Check sheet for the modelled part. Datum: model origin and axes. Units: mm. Face numbers are marked on the shaded views. A direction names the side the tool comes from. Round coordinates to 2 decimals unless told otherwise and drop trailing zeros. Write each loop counter-clockwise with the first axis right and the second up, starting at its lowest first coordinate (ties: lowest second). Pieces come first, ordered by that corner, then holes.
Item 1: Set-up check for the marked faces 1 and 2: record each of +Z, -Z, +X, -X, +Y, -Y from which the full face is reachable in a straight line by a thin tool's end or side.
Item 2: Release check for a two-part mould opening along Z. For the marked faces 3, 4 and 5 record: pulls with the +Z half, pulls with the -Z half, needs draft (parallel to the pull), parting line crosses it, or undercut.
Item 3: Section check B-B, the plane y = 182. Record the cut outline in (x, z), plus the area to 3 significant figures.
Item 4: Material ranges on line 1 along Y through (x, z) = (242.5, 232); line 2 along X through (y, z) = (-184, 194); line 3 along Z through (x, y) = (193.5, 17), recorded low to high.
Item 5: Section check A-A, the plane z = 388.5. State how many separate pieces and enclosed holes the cut face has, plus the area to 3 significant figures.
Item 6: Depth check by flat-ended pin: pin 1 (5 mm diameter, centred on x = 107, y = 40.5, fed in from -Z). Enter the tip coordinate at first touch or a pass-through.
Item 7: Section check C-C, the plane x = 253.5. Record the cut outline in (y, z).
from build123d import *

# Parameters (mm, degrees)
F0_W      = 600
F0_H      = 900
F1_DEPTH  = 500
F2_W      = 475
F2_H      = 150
F3_DEPTH  = 1705
F4_W      = 475
F4_H      = 280
F5_DEPTH  = 846
F6_W      = 100
F6_H      = 500
F7_DEPTH  = 63
F8_DEPTH  = 63
F9_DEPTH  = 63
F10_DEPTH = 63
F11_DEPTH = 63
F13_W     = 100
F13_H     = 500
F14_DEPTH = 63
F15_DEPTH = 63
F16_DEPTH = 63


with BuildPart() as f1:
    # F0 (on Top) → F1 (new body)
    with BuildSketch(Plane.XY):
        Rectangle(F0_W, F0_H)
    extrude(amount=F1_DEPTH)

    # F2 (on face) → F3 (cut)
    with BuildSketch(Plane.XZ.offset(450)):
        with Locations((0, 75)):
            Rectangle(F2_W, F2_H)
    extrude(amount=-F3_DEPTH, mode=Mode.SUBTRACT)

    # F4 (on face) → F5 (cut)
    with BuildSketch(Plane.XZ.offset(450)):
        with Locations((0, 330)):
            Rectangle(F4_W, F4_H)
    extrude(amount=-F5_DEPTH, mode=Mode.SUBTRACT)

    # F6 (on face) → F7 (cut)
    with BuildSketch(Plane.YZ.offset(300)):
        with Locations((-25, 250)):
            Rectangle(F6_W, F6_H)
    extrude(amount=-F7_DEPTH, mode=Mode.SUBTRACT)

    # F8 (add): a face of the model
    f8_faces = [f1.faces().sort_by_distance(p)[0] for p in [
        (237, -25, 485),
    ]]
    extrude(f8_faces, amount=F8_DEPTH)

    # F9 (add): a face of the model
    f9_faces = [f1.faces().sort_by_distance(p)[0] for p in [
        (237, -25, 170),
    ]]
    extrude(f9_faces, amount=F9_DEPTH)

    # F6 (on face) → F10 (cut)
    with BuildSketch(Plane.YZ.offset(300)):
        with Locations((325, 250)):
            Rectangle(F6_W, F6_H)
        with Locations((150, 250)):
            Rectangle(F6_W, F6_H)
        with Locations((-25, 250)):
            Rectangle(F6_W, F6_H)
    extrude(amount=-F10_DEPTH, mode=Mode.SUBTRACT)

    # F11 (add): faces of the model
    f11_faces = [f1.faces().sort_by_distance(p)[0] for p in [
        (237, -25, 485),
        (237, 150, 485),
        (237, 325, 485),
        (237, 325, 170),
        (237, 150, 170),
        (237, -25, 170),
    ]]
    extrude(f11_faces, amount=F11_DEPTH)

    # F13 (on face) → F14 (cut)
    with BuildSketch(Plane(origin=(-300, 0, 0), x_dir=(0, -1, 0), z_dir=(-1, 0, 0))):
        with Locations((-325, 250)):
            Rectangle(F13_W, F13_H)
        with Locations((-150, 250)):
            Rectangle(F13_W, F13_H)
        with Locations((25, 250)):
            Rectangle(F13_W, F13_H)
    extrude(amount=-F14_DEPTH, mode=Mode.SUBTRACT)

    # F15 (add): faces of the model
    f15_faces = [f1.faces().sort_by_distance(p)[0] for p in [
        (-237, 325, 485),
        (-237, 150, 485),
        (-237, -25, 485),
    ]]
    extrude(f15_faces, amount=F15_DEPTH)

    # F16 (add): faces of the model
    f16_faces = [f1.faces().sort_by_distance(p)[0] for p in [
        (-237, 325, 170),
        (-237, 150, 170),
        (-237, -25, 170),
    ]]
    extrude(f16_faces, amount=F16_DEPTH)


solid = f1.part
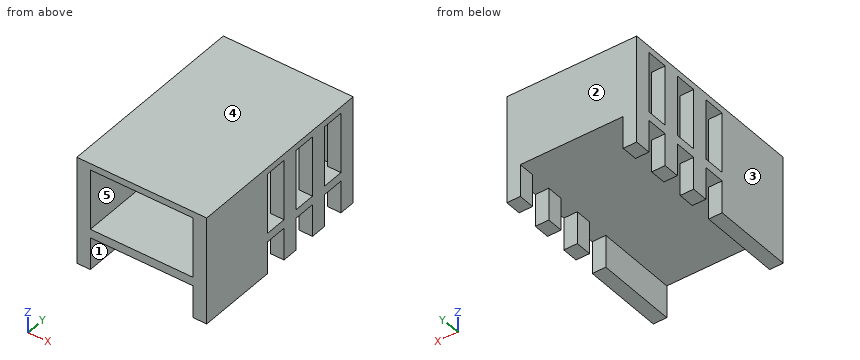
Values found:
1. face 1: -Z, +Y, -Y
1. face 2: +Z, -Z, +X, -X, +Y
2. face 3: needs draft
2. face 4: pulls with the +Z half
2. face 5: undercut
3. outline: (-300, 150) - (300, 150) - (300, 190) - (-300, 190) - close; (-300, 470) - (300, 470) - (300, 500) - (-300, 500) - close
3. area: 42,000 mm2
4. line 1: y = -450 to -75, 25 to 100, 200 to 275, 375 to 450
4. line 2: x = -300 to -237.5, 237.5 to 300
4. line 3: z = 150 to 190, 470 to 500
5. separate pieces: 7
5. enclosed holes: 0
5. area: 101,000 mm2
6. pin 1: stops at z = 150
7. outline: (-450, 0) - (-75, 0) - (-75, 150) - (25, 150) - (25, 0) - (100, 0) - (100, 150) - (200, 150) - (200, 0) - (275, 0) - (275, 150) - (375, 150) - (375, 0) - (450, 0) - (450, 500) - (-450, 500) - close; hole (-75, 190) - (25, 190) - (25, 470) - (-75, 470) - close; hole (100, 190) - (200, 190) - (200, 470) - (100, 470) - close; hole (275, 190) - (375, 190) - (375, 470) - (275, 470) - close
